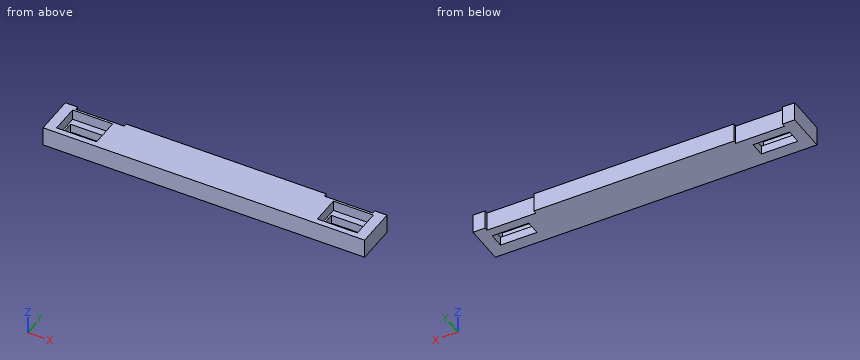
from build123d import *

# Parameters (mm, degrees)
F0_W     = 23
F0_H     = 16.5
F1_DEPTH = 11
F0_W_2   = 21
F0_H_2   = 8.5
F2_DEPTH = 5


with BuildPart() as f1:
    # F0 (on Top) → F1 (new body)
    with BuildSketch(Plane.XY):
        Polygon((-85.5, 11.5), (-92.5, 11.5), (-92.5, -11.5), (92.5, -11.5), (92.5, 11.5), (85.5, 11.5), (85.5, 9.5), (57.5, 9.5), (57.5, 11.5), (-57.5, 11.5), (-57.5, 9.5), (-85.5, 9.5), align=None)
        with Locations((-75, 0)):
            Rectangle(F0_W, F0_H, mode=Mode.SUBTRACT)
        with Locations((75, 0)):
            Rectangle(F0_W, F0_H, mode=Mode.SUBTRACT)
    extrude(amount=F1_DEPTH)

    # F0 (on Top) → F2 (join)
    with BuildSketch(Plane.XY):
        Polygon((-85.5, 11.5), (-92.5, 11.5), (-92.5, -11.5), (92.5, -11.5), (92.5, 11.5), (85.5, 11.5), (85.5, 9.5), (57.5, 9.5), (57.5, 11.5), (-57.5, 11.5), (-57.5, 9.5), (-85.5, 9.5), align=None)
        with Locations((-75, 0)):
            Rectangle(F0_W, F0_H, mode=Mode.SUBTRACT)
        with Locations((75, 0)):
            Rectangle(F0_W, F0_H, mode=Mode.SUBTRACT)
        with Locations((75, 0)):
            Rectangle(F0_W, F0_H)
        with Locations((75, 0)):
            Rectangle(F0_W_2, F0_H_2, mode=Mode.SUBTRACT)
        with Locations((-75, 0)):
            Rectangle(F0_W, F0_H)
        with Locations((-75, 0)):
            Rectangle(F0_W_2, F0_H_2, mode=Mode.SUBTRACT)
    extrude(amount=F2_DEPTH)


solid = f1.part
CAD build for the part. Positions are in the model's coordinates, mm. Round coordinates to 2 decimals unless told otherwise and drop trailing zeros. Write each loop counter-clockwise with the first axis right and the second up, starting at its lowest first coordinate (ties: lowest second). Pieces come first, ordered by that corner, then holes. Notation, with made-up numbers: M 2,49.25 L 18,49.25 A12 cw 18,60.25 Z; hole C 59.25,-4 d6. An arc over 180 degrees is marked long. Use a Markdown table: item, result. Add a question column.
1. Slice it at A-A on z = 7. Give the cut face in (x, y), then the cut area to 3 significant figures.
2. Slice it at C-C on x = -61.5. Give the cut face in (y, z), then the cut area to 3 significant figures.
3. Drill centre lines: probe 1 along X at (y, z) = (-5.5, 6.25); probe 2 along X at (y, z) = (1, 0.75); probe 3 along Y at (x, z) = (-77, 1.5). Where is each one in solid material? Low to high.
4. Slice it at B-B on x = 81. Give the cut face in (y, z).
5. Flat gauge pins, fed straight in: P1, Ø4, axis at x = -80, z = 3, coming from the +Y side; P2, Ø10, axis at x = -70, y = 0.5, coming from the +Z side. Where does each tip first touch, or does it go through?
Reply:
| question | item | result |
|---|---|---|
| 1 | outline | M -92.5,-11.5 L 92.5,-11.5 L 92.5,11.5 L 85.5,11.5 L 85.5,9.5 L 57.5,9.5 L 57.5,11.5 L -57.5,11.5 L -57.5,9.5 L -85.5,9.5 L -85.5,11.5 L -92.5,11.5 Z; hole M -86.5,-8.25 L -63.5,-8.25 L -63.5,8.25 L -86.5,8.25 Z; hole M 63.5,-8.25 L 86.5,-8.25 L 86.5,8.25 L 63.5,8.25 Z |
| 1 | area | 3,380 mm^2 |
| 2 | outline | M -11.5,0 L 9.5,0 L 9.5,11 L -11.5,11 Z |
| 2 | area | 231 mm^2 |
| 3 | probe 1 | x = -92.5 to -86.5, -63.5 to 63.5, 86.5 to 92.5 |
| 3 | probe 2 | x = -92.5 to -85.5, -64.5 to 64.5, 85.5 to 92.5 |
| 3 | probe 3 | y = -11.5 to -4.25, 4.25 to 9.5 |
| 4 | outline | M -11.5,0 L -4.25,0 L -4.25,5 L -8.25,5 L -8.25,11 L -11.5,11 Z; M 4.25,0 L 9.5,0 L 9.5,11 L 8.25,11 L 8.25,5 L 4.25,5 Z |
| 5 | P1 | stops at y = 9.5 |
| 5 | P2 | stops at z = 5 |
